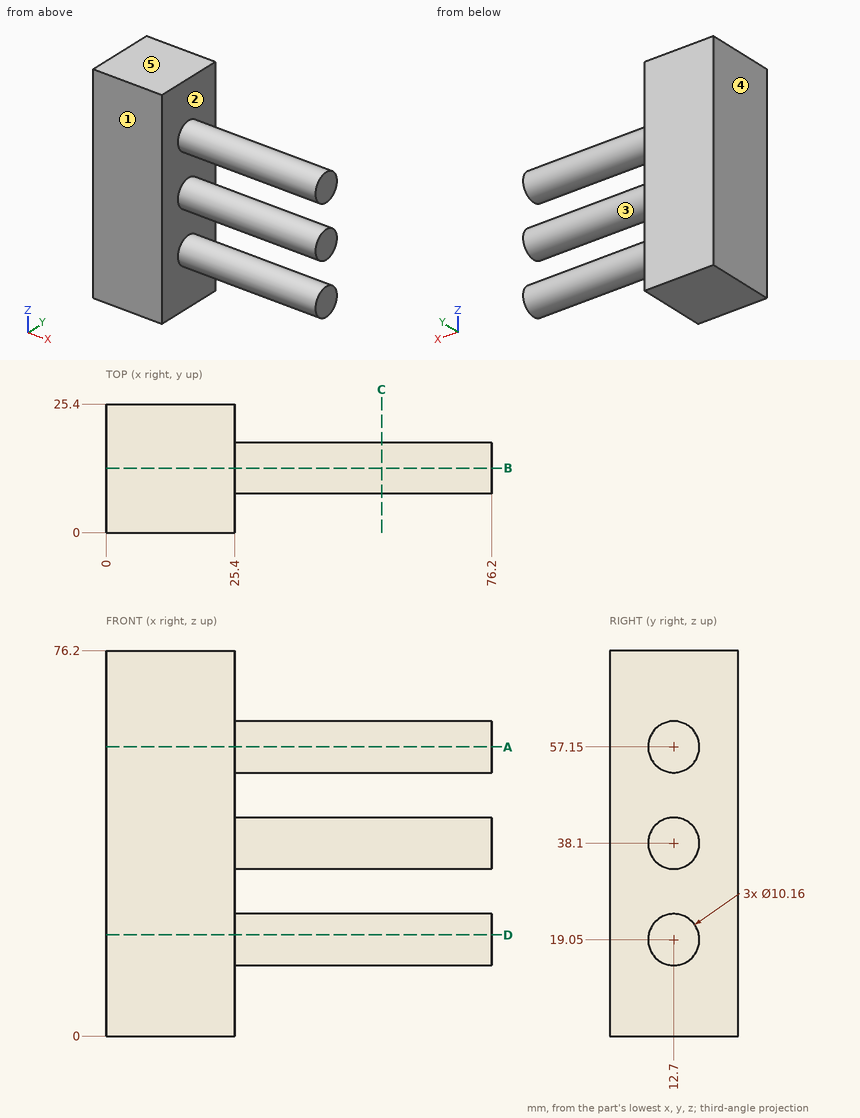
Input: dimensioned drawing with shaded views. Units: mm. Origin: part minimum x, y, z. A direction names the side the tool comes from. Coordinates: 2 decimals unless noted, no trailing zeros. Loops run counter-clockwise (first coordinate to the right, second up) from the corner with the lowest first, then second, coordinate; pieces in that order, holes last. Notation, with made-up numbers: M 78,-13 L 102,-13 A21 ccw 102,0 Z; hole C 62.5,8.5 d2. An arc over 180 degrees is marked long. Use a Markdown table: item, result. Add a question column.
Q1. Access query for the marked faces 1 and 2. Directions: +Z, -Z, +X, -X, +Y, -Y. A direction counts if a zero-diameter tool reaches every point of the face in a straight line with its end or side. Return the directions, or none.
Q2. Material intervals for L1, parallel to Z at x = 50.5, y = 15.5; L2, parallel to X at y = 24, z = 46; L3, parallel to Z at x = 28, y = 16, sorted ascending.
Q3. Draft query along Z for the marked faces 3, 4 and 5. Return one class per face: pulls with the +Z half, pulls with the -Z half, needs draft (parallel to the pull), parting line crosses it, or undercut.
Q4. First-contact query: pin 1 (1 mm diameter, centred on x = 47.5, y = 10, fed in from +Z); pin 2 (6 mm diameter, centred on x = 64.5, z = 13, fed in from -Y); pin 3 (6 mm diameter, centred on y = 3.5, z = 33, fed in from +X). Flat tips, straight axial feed; report the tip coordinate or a pass-through.
Q5. Section query B-B, the plane y = 12.7. Return loops of the section in (x, z).
Q6. Section query A-A, the plane z = 57.15. Return loops of the section in (x, y).
Q7. Section query D-D, the plane z = 20. Return loops of the section in (x, y), and give its area (3 significant figures).
Q8. Section query C-C, the plane x = 54.5. Return loops of the section in (y, z).
Result:
| question | item | result |
|---|---|---|
| 1 | face 1 | +Z, -Z, +X, -X, -Y |
| 1 | face 2 | +X |
| 2 | L1 | z = 14.81 to 23.29, 33.86 to 42.34, 52.91 to 61.39 |
| 2 | L2 | x = 0 to 25.4 |
| 2 | L3 | z = 15.19 to 22.91, 34.24 to 41.96, 53.29 to 61.01 |
| 3 | face 3 | undercut |
| 3 | face 4 | needs draft |
| 3 | face 5 | pulls with the +Z half |
| 4 | pin 1 | stops at z = 61.73 |
| 4 | pin 2 | stops at y = 8.64 |
| 4 | pin 3 | stops at x = 25.4 |
| 5 | outline | M 0,0 L 25.4,0 L 25.4,13.97 L 76.2,13.97 L 76.2,24.13 L 25.4,24.13 L 25.4,33.02 L 76.2,33.02 L 76.2,43.18 L 25.4,43.18 L 25.4,52.07 L 76.2,52.07 L 76.2,62.23 L 25.4,62.23 L 25.4,76.2 L 0,76.2 Z |
| 6 | outline | M 0,0 L 25.4,0 L 25.4,7.62 L 76.2,7.62 L 76.2,17.78 L 25.4,17.78 L 25.4,25.4 L 0,25.4 Z |
| 7 | outline | M 0,0 L 25.4,0 L 25.4,7.71 L 76.2,7.71 L 76.2,17.69 L 25.4,17.69 L 25.4,25.4 L 0,25.4 Z |
| 7 | area | 1,150 mm2 |
| 8 | outline | C 12.7,19.05 d10.16; C 12.7,38.1 d10.16; C 12.7,57.15 d10.16 |
